Check sheet for the drawn part. Datum: minimum x, y, z corner. Units: mm. A direction names the side the tool comes from. Round coordinates to 2 decimals unless told otherwise and drop trailing zeros. Write each loop counter-clockwise with the first axis right and the second up, starting at its lowest first coordinate (ties: lowest second). Pieces come first, ordered by that corner, then holes.
Item 1: Cross-section at A-A on z = 7. Enter the section's corners in (x, y).
Item 2: Cross-section at B-B on y = 29.5. Enter the section's corners in (x, z), plus the area to 3 significant figures.
Item 3: Release check for a two-part mould opening along X. For the marked faces 1, 2, 3 and 4 record: +X half, -X half, draft (parallel to the pull), parting line (faces both ways), or undercut.
Item 4: Material ranges on line 1 (X direction, y = 7.5, z = 24.5); line 2 (Z direction, x = 43, y = 3); line 3 (X direction, y = 38, z = 21.5), recorded low to high.
Item 5: Tool access check on the marked faces 5, 6 and 7. Record the directions out of +Z, -Z, +X, -X, +Y, -Y that give a thin tool (end or side, any length) a straight path to the whole face; none if there is none.
Item 6: Go/stop test with flat-tipped pins: pin 1 Ø6 at (x, z) = (17, 21) entering from +Y; pin 2 Ø11 at (y, z) = (7.5, 37) entering from +X; pin 3 Ø15.5 at (x, y) = (8.5, 35.5) entering from +Z; pin 4 Ø1 at (x, z) = (55, 15.5) entering from -Y. Record where each tip stops, or that it passes through.
Item 7: Cross-section at D-D on y = 34. Enter the section's corners in (x, z), plus the area to 3 significant figures.
Item 8: Cross-section at C-C on z = 34. Enter the section's corners in (x, y).
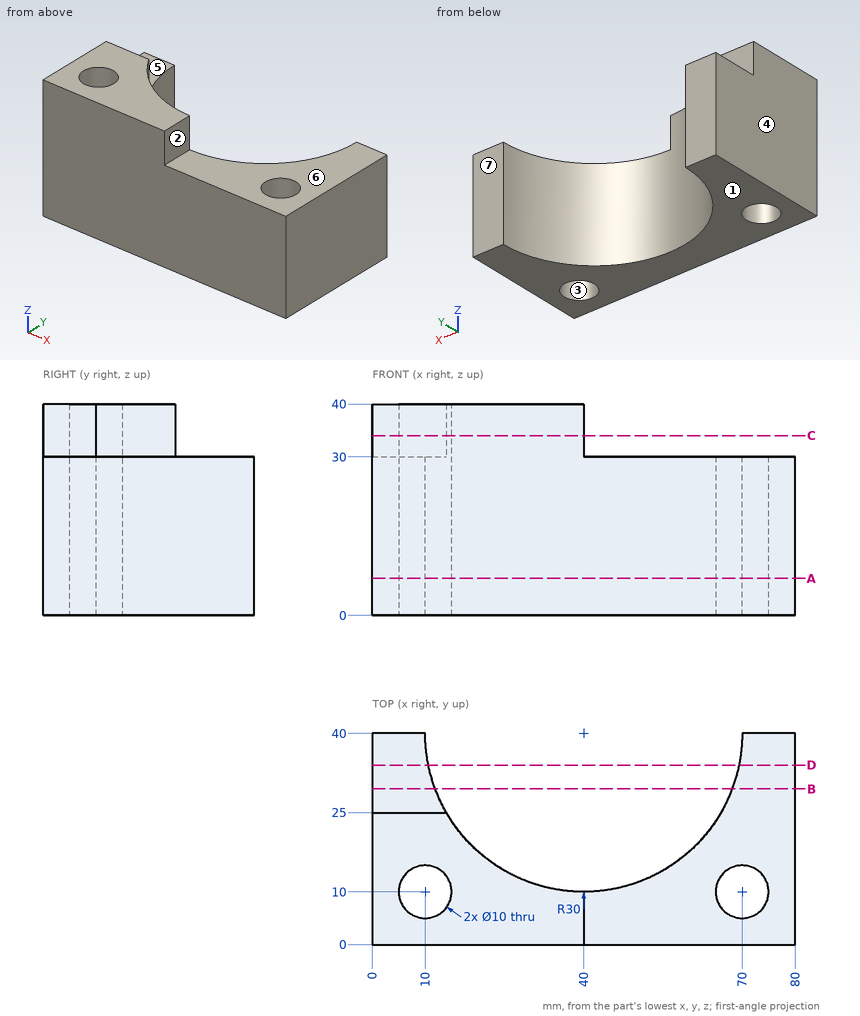
Response values:
1. outline: (0, 0) - (80, 0) - (80, 40) - (70, 40) arc R30 cw to (10, 40) - (0, 40) - close; hole circle Ø10 at (10, 10); hole circle Ø10 at (70, 10)
2. outline: (0, 0) - (11.9, 0) - (11.9, 30) - (0, 30) - close; (68.1, 0) - (80, 0) - (80, 30) - (68.1, 30) - close
2. area: 714 mm2
3. face 1: draft
3. face 2: +X half
3. face 3: undercut
3. face 4: -X half
4. line 1: x = 0 to 5.67, 14.33 to 65.67, 74.33 to 80
4. line 2: z = 0 to 30
4. line 3: x = 0 to 10.07, 69.93 to 80
5. face 5: +Z, +X, -X, +Y
5. face 6: +Z, +X, +Y, -Y
5. face 7: +Z, -Z, +X, -X, +Y
6. pin 1: stops at y = 25.03
6. pin 2: stops at x = 40
6. pin 3: stops at z = 30
6. pin 4: stops at y = 0
7. outline: (0, 0) - (10.61, 0) - (10.61, 30) - (0, 30) - close; (69.39, 0) - (80, 0) - (80, 30) - (69.39, 30) - close
7. area: 636 mm2
8. outline: (0, 0) - (40, 0) - (40, 10) arc R30 cw to (14.02, 25) - (0, 25) - close; hole circle Ø10 at (10, 10)
